Model file for the job. Use its own axes, mm. Face numbers are marked on the shaded views. A direction names the side the tool comes from. Round coordinates to 2 decimals unless told otherwise and drop trailing zeros. Loops run counter-clockwise (first coordinate to the right, second up) from the corner with the lowest first, then second, coordinate; pieces in that order, holes last.
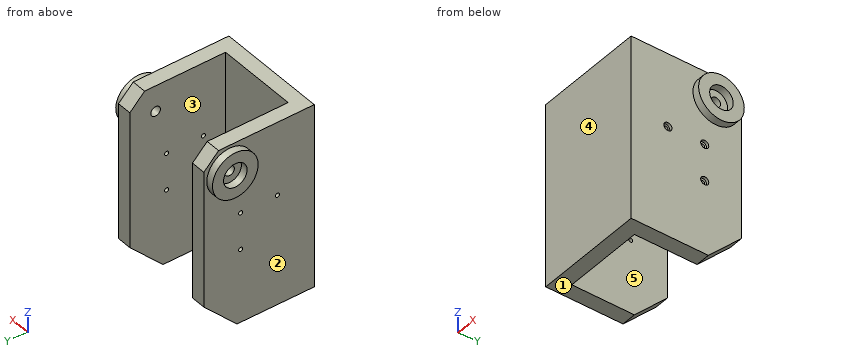
from build123d import *

# Parameters (mm, degrees)
SALIENTE_EXTRUIR1_DEPTH                              = 125
CROQUIS2_R                                           = 31
CROQUIS2_R_2                                         = 16
SALIENTE_EXTRUIR2_DEPTH                              = 10
CROQUIS4_R                                           = 6.5
CORTAR_EXTRUIR2_DEPTH                                = 161
CHAFL_N2_SIZE                                        = 20
CHAFL_N3_SIZE                                        = 45
REFRENTADO_PARA_TORNILLO_CON_CABEZA_TRON_D           = 5.5
REFRENTADO_PARA_TORNILLO_CON_CABEZA_TRON_CBORE_D     = 11
REFRENTADO_PARA_TORNILLO_CON_CABEZA_TRON_CBORE_DEPTH = 3.7


with BuildPart() as part:
    # Croquis1 → Saliente-Extruir1 (new body, symmetric)
    with BuildSketch(Plane.XY):
        Polygon((-55, 130), (-55, 0), (55, 0), (55, 130), (75, 130), (75, -20), (-75, -20), (-75, 130), align=None)
    extrude(amount=SALIENTE_EXTRUIR1_DEPTH, both=True)

    # Croquis2 → Saliente-Extruir2 (add)
    with BuildSketch(Plane(origin=(75, 0, 0), x_dir=(0, 0, -1), z_dir=(1, 0, 0))):
        with Locations(Location((-90, 95, 0), (0, 0, 180))):  # turned: the seam where the file's is
            Circle(CROQUIS2_R)
        with Locations((-90, 95)):
            Circle(CROQUIS2_R_2, mode=Mode.SUBTRACT)
    saliente_extruir2 = extrude(amount=SALIENTE_EXTRUIR2_DEPTH)

    # Simetría1: Saliente-Extruir2 across plane
    add(saliente_extruir2.mirror(Plane(origin=(0, 0, 0), x_dir=(0, 0, 1), z_dir=(1, 0, 0))))

    # Croquis4 → Cortar-Extruir2 (cut, through all)
    with BuildSketch(Plane(origin=(75, 0, 0), x_dir=(0, 0, -1), z_dir=(1, 0, 0))):
        with Locations(Location((-90, 95, 0), (0, 0, 90))):  # turned: the seam where the file's is
            Circle(CROQUIS4_R)
    extrude(amount=-CORTAR_EXTRUIR2_DEPTH, mode=Mode.SUBTRACT)

    # Chaflán2
    chafl_n2_edges = [part.edges().sort_by_distance(p)[0] for p in [
        (65, 130, 125),
        (-65, 130, 125),
    ]]
    chamfer(chafl_n2_edges, length=CHAFL_N2_SIZE)

    # Chaflán3
    chafl_n3_edges = [part.edges().sort_by_distance(p)[0] for p in [
        (-65, 130, -125),
        (65, 130, -125),
    ]]
    chamfer(chafl_n3_edges, length=CHAFL_N3_SIZE)

    # Refrentado para tornillo con cabeza troncocónica de M51 (through all)
    with Locations(Plane(origin=(75, 80, 25), x_dir=(0, 0, 1), z_dir=(1, 0, 0))):
        with Locations((0, 0), (-50, 0), (0, 50)):
            CounterBoreHole(REFRENTADO_PARA_TORNILLO_CON_CABEZA_TRON_D / 2, REFRENTADO_PARA_TORNILLO_CON_CABEZA_TRON_CBORE_D / 2, REFRENTADO_PARA_TORNILLO_CON_CABEZA_TRON_CBORE_DEPTH)


solid = part.part
Q1. Slice it at A-A on y = 30. Give the cut face in (x, z).
Q2. Tool access for the marked faces 4 and 5: list every direction of +Z, -Z, +X, -X, +Y, -Y with a clear straight run to the whole face (end or side of a thin tool).
Q3. Slice it at B-B on z = 25. State how many separate pieces and enclosed holes the cut face has, plus the area to 3 significant figures.
Q4. Probe line 1 (Y direction, x = 72.85, z = 25); line 2 (Z direction, x = -67, y = 80); line 3 (Y direction, x = -65.75, z = 25). List the from-to ranges inside material, lowest first.
Q5. Flat gauge pins, fed straight in: P1, Ø7, axis at y = 30, z = 25, coming from the +X side; P2, Ø9.5, axis at y = 98.5, z = 82, coming from the +X side; P3, Ø10, axis at x = -18.5, z = 99.5, coming from the +Y side. Where does each tip first touch, or does it go through?
Q6. Slice it at D-D on x = -71. Give the cut face in (y, z).
Q7. Pull direction X, two halves, no side cores. Call the marked faces 1, 2 and 3: pulls with the +X half, pulls with the -X half, needs draft (parallel to the pull), parting line crosses it, or undercut.
Q8. Slice it at C-C on z = -25. Give the cut face in (x, y).
Reply:
1. outline: (-75, -125) - (-55, -125) - (-55, 22.25) - (-75, 22.25) - close; (-75, 27.75) - (-55, 27.75) - (-55, 125) - (-75, 125) - close; (55, -125) - (75, -125) - (75, 19.5) - (71.3, 19.5) - (71.3, 22.25) - (55, 22.25) - close; (55, 27.75) - (71.3, 27.75) - (71.3, 30.5) - (75, 30.5) - (75, 125) - (55, 125) - close
2. face 4: +Z, -Z, +X, -X, -Y
2. face 5: +Z, -Z, +Y
3. separate pieces: 5
3. enclosed holes: 0
3. area: 7,720 mm2
4. line 1: y = -20 to 24.5, 35.5 to 74.5, 85.5 to 130
4. line 2: z = -125 to -27.75, -22.25 to 22.25, 27.75 to 125
4. line 3: y = -20 to 27.25, 32.75 to 77.25, 82.75 to 130
5. P1: stops at x = 71.3
5. P2: stops at x = 75
5. P3: stops at y = 0
6. outline: (-20, -125) - (85, -125) - (130, -80) - (130, 105) - (110, 125) - (-20, 125) - close; hole circle Ø5.5 at (30, 25); hole circle Ø5.5 at (80, -25); hole circle Ø5.5 at (80, 25); hole circle Ø13 at (95, 90)
7. face 1: needs draft
7. face 2: pulls with the -X half
7. face 3: undercut
8. outline: (-75, -20) - (75, -20) - (75, 74.5) - (71.3, 74.5) - (71.3, 77.25) - (55, 77.25) - (55, 0) - (-55, 0) - (-55, 77.25) - (-75, 77.25) - close; (-75, 82.75) - (-55, 82.75) - (-55, 130) - (-75, 130) - close; (55, 82.75) - (71.3, 82.75) - (71.3, 85.5) - (75, 85.5) - (75, 130) - (55, 130) - close
